from build123d import *

# Parameters (mm, degrees)
BOSS_EXTRUDE1_DEPTH = 3


with BuildPart() as part:
    # Sketch1 → Boss-Extrude1 (new body)
    with BuildSketch(Plane(origin=(0, 0, 0), x_dir=(1, 0, 0), z_dir=(0, 1, 0))):
        Polygon((22.079481216, 3.028725772), (16.079481216, 3.028725772), (16.079481216, 9.028725772), (0.079481216, 9.028725772), (0.079481216, 3.028725772), (-5.920518784, 3.028725772), (6.579481216, -11.971274228), (6.579481216, -8.971274228), (9.579481216, -8.971274228), (9.579481216, -11.971274228), align=None)
        Polygon((15.674356378, 0.028725772), (0.484606054, 0.028725772), (5.484606054, -5.971274228), (10.674356378, -5.971274228), align=None, mode=Mode.SUBTRACT)
    extrude(amount=BOSS_EXTRUDE1_DEPTH)


solid = part.part
Geometry check sheet. Reference: the model listing, model coordinates, mm. A direction names the side the tool comes from. Give positions to 0.01 mm unless a question says otherwise; leave off trailing zeros. Order: outer loops, then holes, each group sorted by start corner. A loop starts at its lowest first (then second) coordinate and runs counter-clockwise, first axis right, second up.
1. Sectioned sample at A-A (x = 7). Record the boundary of the cut face in (y, z), then the cut area to 3 significant figures.
Completed:
outline: (0, -9.03) - (3, -9.03) - (3, -0.03) - (0, -0.03) - close; (0, 5.97) - (3, 5.97) - (3, 8.97) - (0, 8.97) - close
area: 36.0 mm2
2. Scan lines: line 1 (X direction, y = 2.35, z = -6.5); line 2 (Z direction, x = 11.75, y = 2.1); line 3 (Z direction, x = 11.5, y = 2). Record each from-to range of solid material in increasing order.
Completed:
line 1: x = 0.08 to 16.08
line 2: z = -9.03 to -0.03, 4.68 to 9.37
line 3: z = -9.03 to -0.03, 4.98 to 9.67
3. Sectioned sample at D-D (x = 17). Record the boundary of the cut face in (y, z).
Completed:
outline: (0, -3.03) - (3, -3.03) - (3, 3.07) - (0, 3.07) - close
4. Depth check by flat-ended pin: pin 1 (0.9 mm diameter, centred on x = 5.5, y = 2, fed in from +Z); pin 2 (0.9 mm diameter, centred on x = -4, y = 1.5, fed in from -Z); pin 3 (1 mm diameter, centred on y = 0.5, z = 8, fed in from +X). Enter the tip coordinate at first touch or a pass-through.
Completed:
pin 1: stops at z = 11.22
pin 2: stops at z = -3.03
pin 3: stops at x = 13.31
5. Sectioned sample at C-C (z = 5.25). Record the boundary of the cut face in (x, y).
Completed:
outline: (0.98, 0) - (4.88, 0) - (4.88, 3) - (0.98, 3) - close; (11.28, 0) - (15.18, 0) - (15.18, 3) - (11.28, 3) - close
6. Draft check along Z on faces 1 (the face through (2.95, 1.48, 2.93)), 2 (the face through (19, 1, -3.029)), 3 (the face through (9.579, 1, 10)). Enter one of: pulls with the +Z half, pulls with the -Z half, needs draft (parallel to the pull), parting line crosses it, or undercut.
Completed:
face 1: undercut
face 2: pulls with the -Z half
face 3: needs draft
7. Access from +Z, -Z, +X, -X, +Y, -Y to the whole of each face (thin tool, end or side, straight path). Record for faces 4 (the face through (-3, 1, -3.029)), 5 (the face through (8, 1, 8.971)), 6 (the face through (13.14, 1.48, 3.01)), 7 (the face through (8, 0, -1)), 8 (the face through (16.079, 1, -6)).
Completed:
face 4: -Z, -X, +Y, -Y
face 5: +Z, +Y, -Y
face 6: +Y, -Y
face 7: +Z, -Z, +X, -X, -Y
face 8: -Z, +X, +Y, -Y
8. Sectioned sample at B-B (y = 1.05). Record the boundary of the cut face in (x, z), then the cut area to 3 significant figures.
Completed:
outline: (-5.92, -3.03) - (0.08, -3.03) - (0.08, -9.03) - (16.08, -9.03) - (16.08, -3.03) - (22.08, -3.03) - (9.58, 11.97) - (9.58, 8.97) - (6.58, 8.97) - (6.58, 11.97) - close; hole (0.48, -0.03) - (15.67, -0.03) - (10.67, 5.97) - (5.48, 5.97) - close
area: 258 mm2
